Here's the drawing with two shaded views (mm, measured from the low corner). I have some questions. Give positions to 0.01 mm unless a question says otherwise; leave off trailing zeros. Order: outer loops, then holes, each group sorted by start corner. A loop starts at its lowest first (then second) coordinate and runs counter-clockwise, first axis right, second up. Notation, with made-up numbers: (-1, 39.25) - (20, 39.25) arc R25 cw to (20, 54.25) - close; hole circle Ø2 at (59, 71.25). An arc over 180 degrees is marked (long way). Use one line per item in the form item = value. Start each with the question number.
1) Suppose I cut it at A-A, the plane x = 63.5. Write out the boundary of the cut face in (y, z), and give its area (3 significant figures).
2) Suppose I cut it at C-C, the plane y = 2.4. Write out the boundary of the cut face in (x, z).
3) Suppose I cut it at D-D, the plane x = 85. Write out the boundary of the cut face in (y, z), and give its area (3 significant figures).
4) Suppose I cut it at B-B, the plane z = 7. Write out the boundary of the cut face in (x, y), and give its area (3 significant figures).
5) Please list where these lines run through material, in increasing order: probe 1 along X at (y, z) = (1.1, 7); probe 2 along Z at (x, y) = (50.5, 0.7); probe 3 along Z at (x, y) = (85, 2).
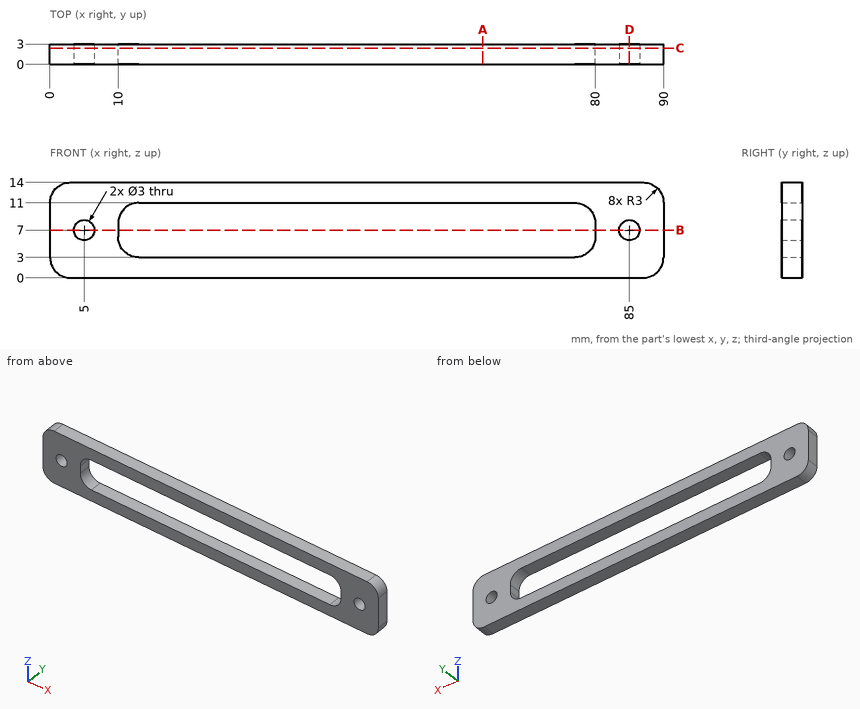
Result sheet:
q1.outline = (0, 0) - (3, 0) - (3, 3) - (0, 3) - close; (0, 11) - (3, 11) - (3, 14) - (0, 14) - close
q1.area = 18.0 mm²
q2.outline = (0, 3) arc R3 ccw to (3, 0) - (87, 0) arc R3 ccw to (90, 3) - (90, 11) arc R3 ccw to (87, 14) - (3, 14) arc R3 ccw to (0, 11) - close; hole circle Ø3 at (5, 7); hole (10, 6) arc R3 ccw to (13, 3) - (77, 3) arc R3 ccw to (80, 6) - (80, 8) arc R3 ccw to (77, 11) - (13, 11) arc R3 ccw to (10, 8) - close; hole circle Ø3 at (85, 7)
q3.outline = (0, 0) - (3, 0) - (3, 5.5) - (0, 5.5) - close; (0, 8.5) - (3, 8.5) - (3, 14) - (0, 14) - close
q3.area = 33.0 mm²
q4.outline = (0, 0) - (3.5, 0) - (3.5, 3) - (0, 3) - close; (6.5, 0) - (10, 0) - (10, 3) - (6.5, 3) - close; (80, 0) - (83.5, 0) - (83.5, 3) - (80, 3) - close; (86.5, 0) - (90, 0) - (90, 3) - (86.5, 3) - close
q4.area = 42.0 mm²
q5.probe_1 = 0 to 3.5, 6.5 to 10, 80 to 83.5, 86.5 to 90
q5.probe_2 = 0 to 3, 11 to 14
q5.probe_3 = 0 to 5.5, 8.5 to 14
